```python
from build123d import *

# Parameters (mm, degrees)
SKETCH1_R               = 45
BOSS_EXTRUDE1_DEPTH     = 15
SKETCH2_R               = 43.5
CUT_EXTRUDE1_DEPTH      = 4.8
SKETCH3_R               = 43.487927738
SKETCH3_R_2             = 38.8
CUT_EXTRUDE2_DEPTH      = 5.4
BOSS_EXTRUDE2_START     = 60
SKETCH4_R               = 45
BOSS_EXTRUDE2_DEPTH     = 60
SKETCH6_R               = 8
CUT_EXTRUDE4_DEPTH      = 71
CUT_EXTRUDE6_DEPTH      = 66
SKETCH11_W              = 26.5
SKETCH11_H              = 38.6
SKETCH11_W_2            = 25.5
SKETCH11_H_2            = 37.6
BOSS_EXTRUDE3_DEPTH     = 3
SKETCH12_W              = 10
SKETCH12_H              = 14
CUT_EXTRUDE_THIN1_DEPTH = 10
SKETCH13_R              = 2
CUT_EXTRUDE7_DEPTH      = 10


with BuildPart() as part:
    # Sketch1 → Boss-Extrude1 (new body)
    with BuildSketch(Plane(origin=(0, 0, 0), x_dir=(1, 0, 0), z_dir=(0, 1, 0))):
        with Locations(Location((0, 0, 0), (0, 0, 270))):
            Circle(SKETCH1_R)
    extrude(amount=BOSS_EXTRUDE1_DEPTH)

    # Sketch2 → Cut-Extrude1 (cut)
    with BuildSketch(Plane(origin=(0, 15, 0), x_dir=(1, 0, 0), z_dir=(0, 1, 0))):
        with Locations(Location((0, 0, 0), (0, 0, 270))):
            Circle(SKETCH2_R)
    extrude(amount=-CUT_EXTRUDE1_DEPTH, mode=Mode.SUBTRACT)

    # Sketch3 → Cut-Extrude2 (cut)
    with BuildSketch(Plane(origin=(0, 10.2, 0), x_dir=(1, 0, 0), z_dir=(0, 1, 0))):
        with Locations(Location((0, 0, 0), (0, 0, 270))):
            Circle(SKETCH3_R)
        with Locations(Location((0, 0, 0), (0, 0, 270))):
            Circle(SKETCH3_R_2, mode=Mode.SUBTRACT)
    extrude(amount=-CUT_EXTRUDE2_DEPTH, mode=Mode.SUBTRACT)

    # Sketch4 → Boss-Extrude2 (add)
    with BuildSketch(Plane.XZ.offset(BOSS_EXTRUDE2_START)):
        with Locations(Location((0, 0, 0), (0, 0, 270))):
            Circle(SKETCH4_R)
    extrude(amount=-BOSS_EXTRUDE2_DEPTH)

    # Sketch6 → Cut-Extrude4 (cut)
    with BuildSketch(Plane.XZ.offset(60)):
        with Locations(Location((0, 0, 0), (0, 0, 270))):
            Circle(SKETCH6_R)
    extrude(amount=-CUT_EXTRUDE4_DEPTH, mode=Mode.SUBTRACT)

    # Sketch10 → Cut-Extrude6 (cut)
    with BuildSketch(Plane(origin=(0, 10.2, 0), x_dir=(1, 0, 0), z_dir=(0, 1, 0))):
        with BuildLine():
            Line((-33.248157844, 20), (-33.248157844, -20))
            ThreePointArc((-33.248157844, -20), (0, -38.8), (33.248157844, -20))
            Line((33.248157844, -20), (33.248157844, 20))
            ThreePointArc((33.248157844, 20), (0, 38.8), (-33.248157844, 20))
        make_face()
    extrude(amount=-CUT_EXTRUDE6_DEPTH, mode=Mode.SUBTRACT)

    # Sketch11 → Boss-Extrude3 (add)
    with BuildSketch(Plane(origin=(-33.248157844, 0, 0), x_dir=(0, 0, -1), z_dir=(1, 0, 0))):
        with Locations((0, -18.8)):
            Rectangle(SKETCH11_W, SKETCH11_H)
        with Locations((0, -18.8)):
            Rectangle(SKETCH11_W_2, SKETCH11_H_2, mode=Mode.SUBTRACT)
    boss_extrude3 = extrude(amount=BOSS_EXTRUDE3_DEPTH)

    # Mirror1: Boss-Extrude3 across plane
    add(boss_extrude3.mirror(Plane(origin=(0, 0, 0), x_dir=(0, 0, 1), z_dir=(1, 0, 0))))

    # Sketch12 → Cut-Extrude-Thin1 (cut)
    with BuildSketch(Plane(origin=(0, -55.8, 0), x_dir=(1, 0, 0), z_dir=(0, 1, 0))):
        with Locations((-24.509146191, 0)):
            Rectangle(SKETCH12_W, SKETCH12_H)
        with Locations((21.509146191, 0)):
            Rectangle(SKETCH12_W, SKETCH12_H)
    extrude(amount=-CUT_EXTRUDE_THIN1_DEPTH, mode=Mode.SUBTRACT)

    # Sketch13 → Cut-Extrude7 (cut)
    with BuildSketch(Plane.XZ.offset(60)):
        with Locations(Location((0, 35, 0), (0, 0, 270))):
            Circle(SKETCH13_R)
        with Locations(Location((0, -35, 0), (0, 0, 90))):
            Circle(SKETCH13_R)
    extrude(amount=-CUT_EXTRUDE7_DEPTH, mode=Mode.SUBTRACT)


solid = part.part
```
Can you work these out from the model? Positions are in its coordinate system, mm. A direction names the side the tool comes from. Coordinates: 2 decimals unless noted, no trailing zeros. Loops run counter-clockwise (first coordinate to the right, second up) from the corner with the lowest first, then second, coordinate; pieces in that order, holes last. Notation, with made-up numbers: (-28, -6) - (-21, -6) arc R34 ccw to (-21, 30) - close; hole circle Ø4 at (57, 63.25). An arc over 180 degrees is marked (long way). Use a Markdown table: item, result.
Item 1: For faces 1 (the face through (-19.509, -58, 0)), 2 (the face through (32, -19, -13.25)), 3 (the face through (32, -37.6, 0)), which set-ups out of +Z, -Z, +X, -X, +Y, -Y let a thin tool reach every point of the face, with its end or its side?
Numbers:
| item | result |
|---|---|
| face 1 | +Y, -Y |
| face 2 | +Y |
| face 3 | none |
Item 2: Will these pins go through, and if not, where does the flat tip stop? pin 1 (6 mm diameter, centred on y = -9, z = 3.5, fed in from -X); pin 2 (1 mm diameter, centred on x = 33.5, y = -41.5, fed in from -Z); pin 3 (8 mm diameter, centred on y = 3.5, z = 20, fed in from -X); pin 4 (3 mm diameter, centred on x = 0, z = 35, fed in from -Y).
Numbers:
| item | result |
|---|---|
| pin 1 | stops at x = -45 |
| pin 2 | stops at z = -30.59 |
| pin 3 | stops at x = -42.06 |
| pin 4 | passes through |
Item 3: We'd pull the mould along Z, two halves only. Please class faces 4 (the face through (-0.766, -57.929, 33.153)), 5 (the face through (-0.559, -25.076, 38.796)), 6 (the face through (1, -60, -9)): released by +Z, released by -Z, zero draft, split by the parting line, or undercut.
Numbers:
| item | result |
|---|---|
| face 4 | undercut |
| face 5 | undercut |
| face 6 | zero draft |
Item 4: If I drill on probe 1 along X at (y, z) = (13.15, 0); probe 2 along X at (y, z) = (-56.85, 0); probe 3 along Y at (x, z) = (-26, 25.5), over which ranges is the centre line in solid material (lowest first)? Write a range as from..to.
Numbers:
| item | result |
|---|---|
| probe 1 | x = -45..-43.5, 43.5..45 |
| probe 2 | x = -45..-29.51, -19.51..-8, 8..16.51, 26.51..45 |
| probe 3 | y = -60..-55.8 |
Item 5: I want a section at B-B on x = 0. Give the number of separate pieces and of enclosed holes in the cut face, and give its area (3 significant figures).
Numbers:
| item | result |
|---|---|
| separate pieces | 4 |
| enclosed holes | 0 |
| area | 1,060 mm2 |
Item 6: I want a section at A-A on y = -45. Please give me the cut outline in (x, z).
Numbers:
| item | result |
|---|---|
| outline | circle Ø90 at (0, 0); hole (-33.25, -20) arc R38.8 ccw to (33.25, -20) - (33.25, 20) arc R38.8 ccw to (-33.25, 20) - close |
